Read the model definition and answer for the solid it produces. Units are mm, in the model's axes. Face numbers are marked on the shaded views. A direction names the side the tool comes from. Coordinates: 2 decimals unless noted, no trailing zeros. Write each loop counter-clockwise with the first axis right and the second up, starting at its lowest first coordinate (ties: lowest second). Pieces come first, ordered by that corner, then holes.
(1) The part is cut by section A-A, the plane y = 22.6. Determine the outline of the cut face in (x, z).
(2) The part is cut by section D-D, the plane z = 37. Determine the outline of the cut face in (x, y).
(3) Determine the mould class of the marked faces 4, 5 and 6 for opening direction X: pulls with the +X half, pulls with the -X half, needs draft (parallel to the pull), parting line crosses it, or undercut.
(4) Straight lines are drawn through the part: line 1 along Y through (x, z) = (7, 13); line 2 along Z through (x, y) = (10.75, -22.6); line 3 along Y through (x, z) = (10.25, 34.5). For each, find the intervals that lie inside material, in ascending order.
(5) Given pin 1 (1.5 mm diameter, centred on y = 1.5, z = 11, fed in from -X); pin 2 (1 mm diameter, centred on x = 18.5, y = 23, fed in from -Z); pin 3 (5 mm diameter, centred on y = -71, z = 11, fed in from +X); pin 4 (1.5 mm diameter, centred on x = 29, z = 28, fed in from +Y), each flat-ended and moving along its own axis, determine where each tip first touches the part or whether it passes through.
(6) Which of the six approach directions +Z, -Z, +X, -X, +Y, -Y give full straight-line access (tool end or side, diameter ignored) to the marked faces 1, 2 and 3?
```python
from build123d import *

# Parameters (mm, degrees)
BOSS_EXTRU_1_DEPTH      = 30
ESQUISSE3_R             = 2.6
ENL_V_MAT_EXTRU_1_DEPTH = 30
ENL_V_MAT_EXTRU_2_DEPTH = 3.5
ESQUISSE6_W             = 16.189542707
ESQUISSE6_H             = 20
BOSS_EXTRU_2_DEPTH      = 27.5
ESQUISSE7_W             = 7.5
ESQUISSE7_H             = 20
BOSS_EXTRU_3_DEPTH      = 12.5
ESQUISSE9_W             = 45
ESQUISSE9_H             = 5.5
ESQUISSE9_R             = 1
ENL_V_MAT_EXTRU_4_DEPTH = 5
ESQUISSE10_R            = 1.5
BOSS_EXTRU_4_DEPTH      = 1.4
CHANFREIN1_SIZE         = 1
ENL_V_MAT_EXTRU_5_DEPTH = 25
ESQUISSE12_W            = 2.7
ESQUISSE12_H            = 20
BOSS_EXTRU_5_DEPTH      = 2
CHANFREIN2_SIZE         = 2
ESQUISSE13_W            = 2.7
ESQUISSE13_H            = 30
BOSS_EXTRU_6_DEPTH      = 2
CHANFREIN3_SIZE         = 2
ENL_V_START             = -12.5
ESQUISSE15_W            = 17
ESQUISSE15_H            = 9.5
ENL_V_MAT_EXTRU_6_DEPTH = 12.5


# Some blends are built 0.0001 mm under size
with BuildPart() as part:
    # Esquisse1 → Boss.-Extru.1 (new body)
    with BuildSketch(Plane.XY):
        with BuildLine():
            Line((4.110457293, 9.444264971), (4.110457293, 30))
            Line((4.110457293, 30), (20.3, 30))
            Line((20.3, 30), (20.3, -81.944264971))
            Line((20.3, -81.944264971), (32.8, -81.944264971))
            Line((32.8, -81.944264971), (32.8, -89.444264971))
            Line((32.8, -89.444264971), (4.110457293, -89.444264971))
            Line((4.110457293, -89.444264971), (4.110457293, -9.444264971))
            ThreePointArc((4.110457293, -9.444264971), (10.3, 0), (4.110457293, 9.444264971))
        make_face()
    extrude(amount=BOSS_EXTRU_1_DEPTH)

    # Esquisse3 → Enlèv. mat.-Extru.1 (cut)
    with BuildSketch(Plane.ZY.offset(-4.110457293)):
        with Locations(Location((15, 22.6, 0), (0, 0, 270))):
            Circle(ESQUISSE3_R)
        with Locations(Location((15, -22.6, 0), (0, 0, 270))):
            Circle(ESQUISSE3_R)
    extrude(amount=-ENL_V_MAT_EXTRU_1_DEPTH, mode=Mode.SUBTRACT)

    # Esquisse4 → Enlèv. mat.-Extru.2 (cut)
    with BuildSketch(Plane(origin=(20.3, 0, 0), x_dir=(0, 0, -1), z_dir=(1, 0, 0))):
        Polygon((-15, -18.443078062), (-18.6, -20.521539031), (-18.6, -24.678460969), (-15, -26.756921938), (-11.4, -24.678460969), (-11.4, -20.521539031), align=None)
        Polygon((-15, 26.756921938), (-18.6, 24.678460969), (-18.6, 20.521539031), (-15, 18.443078062), (-11.4, 20.521539031), (-11.4, 24.678460969), align=None)
    extrude(amount=-ENL_V_MAT_EXTRU_2_DEPTH, mode=Mode.SUBTRACT)

    # Esquisse6 → Boss.-Extru.2 (add)
    with BuildSketch(Plane.XY.offset(30)):
        with Locations((12.205228647, -34.444264971)):
            Rectangle(ESQUISSE6_W, ESQUISSE6_H)
    extrude(amount=BOSS_EXTRU_2_DEPTH)

    # Esquisse7 → Boss.-Extru.3 (add)
    with BuildSketch(Plane(origin=(20.3, 0, 0), x_dir=(0, 0, -1), z_dir=(1, 0, 0))):
        with Locations((-53.75, -34.444264971)):
            Rectangle(ESQUISSE7_W, ESQUISSE7_H)
    extrude(amount=BOSS_EXTRU_3_DEPTH)

    # Esquisse9 → Enlèv. mat.-Extru.4 (cut)
    with BuildSketch(Plane(origin=(20.3, 0, 0), x_dir=(0, 0, -1), z_dir=(1, 0, 0))):
        with Locations((-22.5, -34.444264971)):
            Rectangle(ESQUISSE9_W, ESQUISSE9_H)
        with Locations((-43, -34.444264971)):
            Circle(ESQUISSE9_R, mode=Mode.SUBTRACT)
    extrude(amount=-ENL_V_MAT_EXTRU_4_DEPTH, mode=Mode.SUBTRACT)

    # Esquisse10 → Boss.-Extru.4 (add)
    with BuildSketch(Plane(origin=(20.3, 0, 0), x_dir=(0, 0, -1), z_dir=(1, 0, 0))):
        with Locations((-43, -34.444264971)):
            Circle(ESQUISSE10_R)
    extrude(amount=-BOSS_EXTRU_4_DEPTH)

    # Chanfrein1
    # the kernel refuses this chamfer: 1 mm, written as the material it takes off along each edge
    with BuildSketch(Plane(origin=(18.9, -34.444264971, 43), x_dir=(0, 0, -1), z_dir=(0, -1, 0))) as chanfrein1_piece_1_section:
        Polygon((1.5 - CHANFREIN1_SIZE, 0), (1.5, CHANFREIN1_SIZE), (1.5, 0), align=None)
    chanfrein1_piece_1 = revolve(axis=Axis((18.9, -34.444264971, 43), (1, 0, 0)), mode=Mode.PRIVATE)
    chanfrein1_piece_1 = chanfrein1_piece_1 - Plane(origin=(19.653593842, -34.444264971, 43), x_dir=(0, 0, -1), z_dir=(1, 0, 0)) * Cylinder(1, 7, mode=Mode.PRIVATE)
    add(chanfrein1_piece_1, mode=Mode.SUBTRACT)

    # Esquisse11 → Enlèv. mat.-Extru.5 (cut)
    with BuildSketch(Plane(origin=(0, 0, 0), x_dir=(-1, 0, 0), z_dir=(0, 0, -1))):
        Polygon((-12.110457293, -32.694264971), (-7.110457293, -32.694264971), (-4.850170078, -34.444264971), (-7.110457293, -36.194264971), (-12.110457293, -36.194264971), (-14.370744508, -34.444264971), align=None)
    extrude(amount=-ENL_V_MAT_EXTRU_5_DEPTH, mode=Mode.SUBTRACT)

    # Esquisse12 → Boss.-Extru.5 (add)
    with BuildSketch(Plane(origin=(0, 0, 50), x_dir=(-1, 0, 0), z_dir=(0, 0, -1))):
        with Locations((-31.45, -34.444264971)):
            Rectangle(ESQUISSE12_W, ESQUISSE12_H)
    extrude(amount=BOSS_EXTRU_5_DEPTH)

    # Chanfrein2
    chanfrein2_edges = [part.edges().sort_by_distance(p)[0] for p in [
        (30.1, -34.444264971, 48),
    ]]
    chamfer(chanfrein2_edges, length=CHANFREIN2_SIZE - 0.0001)  # a hair under: the kernel refuses the full size

    # Esquisse13 → Boss.-Extru.6 (add)
    with BuildSketch(Plane(origin=(0, -81.944264971, 0), x_dir=(1, 0, 0), z_dir=(0, 1, 0))):
        with Locations((31.45, -15)):
            Rectangle(ESQUISSE13_W, ESQUISSE13_H)
    extrude(amount=BOSS_EXTRU_6_DEPTH)

    # Chanfrein3
    chanfrein3_edges = [part.edges().sort_by_distance(p)[0] for p in [
        (30.1, -79.944264971, 15),
    ]]
    chamfer(chanfrein3_edges, length=CHANFREIN3_SIZE - 0.0001)  # a hair under: the kernel refuses the full size

    # Esquisse15 → Enlèv. mat.-Extru.6 (cut)
    with BuildSketch(Plane(origin=(32.8, 0, 0), x_dir=(0, 0, -1), z_dir=(1, 0, 0)).offset(ENL_V_START)):
        with Locations((-15, -84.694264971)):
            Rectangle(ESQUISSE15_W, ESQUISSE15_H)
    extrude(amount=ENL_V_MAT_EXTRU_6_DEPTH, mode=Mode.SUBTRACT)


solid = part.part
```
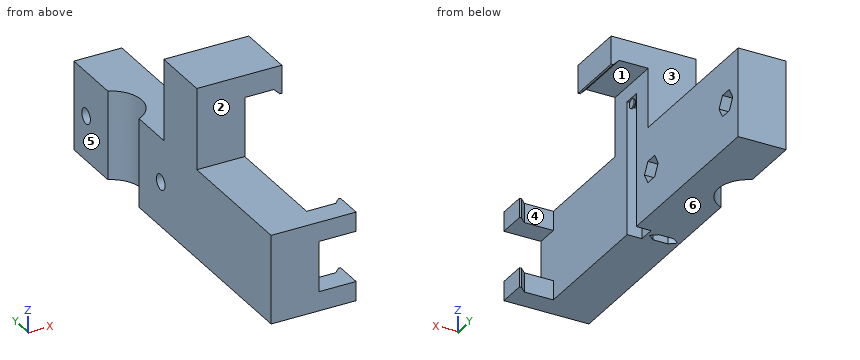
Computed:
1. outline: (4.11, 0) - (20.3, 0) - (20.3, 11.4) - (16.8, 11.4) - (16.8, 12.4) - (4.11, 12.4) - close; (4.11, 17.6) - (16.8, 17.6) - (16.8, 18.6) - (20.3, 18.6) - (20.3, 30) - (4.11, 30) - close
2. outline: (4.11, -44.44) - (20.3, -44.44) - (20.3, -37.19) - (15.3, -37.19) - (15.3, -31.69) - (20.3, -31.69) - (20.3, -24.44) - (4.11, -24.44) - close
3. face 4: undercut
3. face 5: pulls with the -X half
3. face 6: needs draft
4. line 1: y = -89.44 to -36.11, -32.78 to -24.26, -20.94 to -7.56, 7.56 to 20.94, 24.26 to 30
4. line 2: z = 0 to 12.4, 17.6 to 30
4. line 3: y = -44.44 to -24.44
5. pin 1: stops at x = 10.05
5. pin 2: stops at z = 0
5. pin 3: stops at x = 20.3
5. pin 4: stops at y = -81.94
6. face 1: -Z, +Y, -Y
6. face 2: +Z, +X, -X, -Y
6. face 3: +Z, +X, -X, +Y
